The listing builds one solid part. Answer for the finished solid, in the listing's coordinates (mm). Give positions to 0.01 mm unless a question says otherwise; leave off trailing zeros. Order: outer loops, then holes, each group sorted by start corner. A loop starts at its lowest first (then second) coordinate and runs counter-clockwise, first axis right, second up. Notation, with made-up numbers: (-29, -26.75) - (24, -26.75) arc R22 ccw to (24, -3.75) - close; hole circle Ø8 at (57.25, 57.5). An arc over 180 degrees is marked (long way). Answer as a JSON object with one key per item and string values. Group by question number.
Q1. A cutting plane is placed at A-A, the plane y = -27. Give the vertices of the cut face in (x, z), and give its area (3 significant figures).
Q2. A cutting plane is placed at D-D, the plane y = 99.5. Give the vertices of the cut face in (x, z), and give its area (3 significant figures).
Q3. Consider line 1 (Z direction, x = 1.75, y = 104.5); line 2 (Z direction, x = 4.75, y = 79.5); line 3 (Y direction, x = 1.25, z = -1). Determine where each line is inside the solid, lowest interval first.
Q4. A cutting plane is placed at B-B, the plane x = 2. Give the vertices of the cut face in (y, z).
Q5. Given pin 1 (3 mm diameter, centred on x = 3.5, z = -8, fed in from -Y); pin 2 (2 mm diameter, centred on x = 1.5, z = -27.5, fed in from +Y); pin 3 (3 mm diameter, centred on x = 4.5, y = 109, fed in from -Z), each flat-ended and moving along its own axis, determine where each tip first touches the part or whether it passes through.
Q6. A cutting plane is placed at C-C, the plane z = -29.5. Give the vertices of the cut face in (x, y).
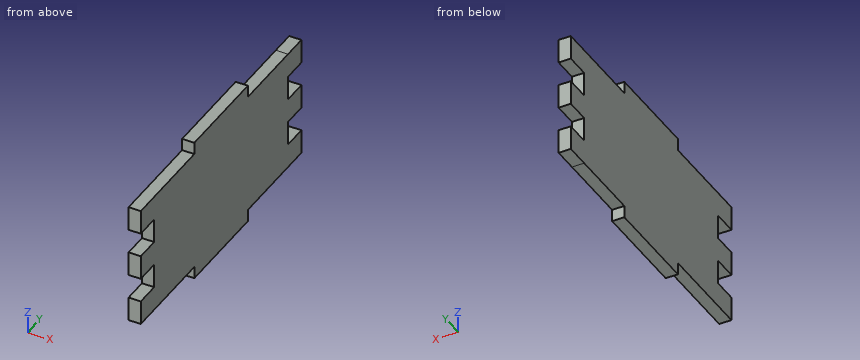
from build123d import *

# Parameters (mm, degrees)
F0_W     = 12.7
F0_H     = 12.7
F0_W_2   = 50.8
F0_H_2   = 6.35
F1_DEPTH = 6.35


# Not quite as in the source:
# - ends of sketch curves that miss each other by under 0.0002 mm in the source are joined


with BuildPart() as f1:
    # F0 (on Right) → F1 (new body)
    with BuildSketch(Plane.YZ):
        with Locations((-31.75, 6.35)):
            Rectangle(F0_W, F0_H)
        Polygon((12.7, 12.7), (-25.4, 12.7), (-25.4, 0), (-25.4, -12.7), (-25.4, -25.4), (-25.4, -38.1), (-25.4, -50.8), (12.7, -50.8), (63.5, -50.8), (101.6, -50.8), (101.6, -38.0999993861), (101.6, -25.3999993861), (101.6, -12.6999993861), (101.6, 6.139e-07), (101.6, 12.7), (63.5, 12.7), align=None)
        with Locations((-31.75, -19.05)):
            Rectangle(F0_W, F0_H)
        with Locations((-31.75, -44.45)):
            Rectangle(F0_W, F0_H)
        with Locations((38.1, -53.975)):
            Rectangle(F0_W_2, F0_H_2)
        with Locations((38.1, 15.875)):
            Rectangle(F0_W_2, F0_H_2)
        with Locations((107.95, 6.3500006139)):
            Rectangle(F0_W, F0_H)
        with Locations((107.95, -19.0499993861)):
            Rectangle(F0_W, F0_H)
        Polygon((114.3, -38.0999993861), (101.6, -38.0999993861), (101.6, -50.8), (114.3, -50.7999993861), align=None)
    extrude(amount=F1_DEPTH)


solid = f1.part
Reply:
{
 "1": {"outline": "(0, -50.8) - (6.35, -50.8) - (6.35, -38.1) - (0, -38.1) - close; (0, -25.4) - (6.35, -25.4) - (6.35, -12.7) - (0, -12.7) - close; (0, 0) - (6.35, 0) - (6.35, 12.7) - (0, 12.7) - close", "area": "242 mm^2"},
 "2": {"outline": "(0, -50.8) - (6.35, -50.8) - (6.35, 12.7) - (0, 12.7) - close", "area": "403 mm^2"},
 "3": {"line 1": "z = -50.8 to -38.1, -25.4 to -12.7, 0 to 12.7", "line 2": "z = -50.8 to 12.7", "line 3": "y = -25.4 to 101.6"},
 "4": {"outline": "(-38.1, -50.8) - (12.7, -50.8) - (12.7, -57.15) - (63.5, -57.15) - (63.5, -50.8) - (114.3, -50.8) - (114.3, -38.1) - (101.6, -38.1) - (101.6, -25.4) - (114.3, -25.4) - (114.3, -12.7) - (101.6, -12.7) - (101.6, 0) - (114.3, 0) - (114.3, 12.7) - (63.5, 12.7) - (63.5, 19.05) - (12.7, 19.05) - (12.7, 12.7) - (-38.1, 12.7) - (-38.1, 0) - (-25.4, 0) - (-25.4, -12.7) - (-38.1, -12.7) - (-38.1, -25.4) - (-25.4, -25.4) - (-25.4, -38.1) - (-38.1, -38.1) - close"},
 "5": {"pin 1": "stops at y = -25.4", "pin 2": "stops at y = 101.6", "pin 3": "stops at z = -50.8"},
 "6": {"outline": "(0, -25.4) - (6.35, -25.4) - (6.35, 101.6) - (0, 101.6) - close"}
}
